For this review, take the finished solid that the model builds, in its own axes (mm). Give positions to 0.01 mm unless a question says otherwise; leave off trailing zeros. Loops run counter-clockwise (first coordinate to the right, second up) from the corner with the lowest first, then second, coordinate; pieces in that order, holes last. Notation, with made-up numbers: (-26.75, 42.25) - (28.25, 42.25) arc R16 cw to (28.25, 49.25) - close; hole circle Ø7 at (87, 82.25). An arc over 180 degrees is marked (long way). Put each result on its own line as item: value. Start each with the question number.
from build123d import *

# Parameters (mm, degrees)
SKETCH1_R            = 15
BOSS_EXTRUDE1_DEPTH  = 1.5875
M5_CLEARANCE_HOLE1_D = 5.8
FILLET1_R            = 10


with BuildPart() as part:
    # Sketch1 → Boss-Extrude1 (new body)
    with BuildSketch(Plane.XY):
        with BuildLine():
            Line((-31.721304871, -10.769995549), (-31.721304871, -61.809795549))
            Line((-31.721304871, -61.809795549), (-244.957511762, -61.809795549))
            Line((-244.957511762, -61.809795549), (-244.957511762, 103.169804451))
            Line((-244.957511762, 103.169804451), (335.042488238, 103.169804451))
            Line((335.042488238, 103.169804451), (335.042488238, -61.809795549))
            Line((335.042488238, -61.809795549), (23.278695129, -61.809795549))
            Line((23.278695129, -61.809795549), (23.278695129, -10.769995549))
            ThreePointArc((23.278695129, -10.769995549), (-4.221304871, 16.730004451), (-31.721304871, -10.769995549))
        make_face()
        with Locations((41.778695129, 44.230004451)):
            Circle(SKETCH1_R, mode=Mode.SUBTRACT)
    extrude(amount=BOSS_EXTRUDE1_DEPTH)

    # M5 Clearance Hole1 (through all)
    with Locations(Plane.XY.offset(1.5875)):
        with Locations((-204.957511762, 93.169804451), (-204.957511762, -51.809795549), (88.121775735, -51.809795549), (295.042488238, -51.809795549), (-84.957511762, 93.169804451), (175.042488238, 93.169804451), (295.042488238, 93.169804451)):
            Hole(M5_CLEARANCE_HOLE1_D / 2)

    # Fillet1
    fillet1_edges = [part.edges().sort_by_distance(p)[0] for p in [
        (-244.957511762, 103.169804451, 0.79375),
        (335.042488238, 103.169804451, 0.79375),
        (335.042488238, -61.809795549, 0.79375),
        (23.278695129, -61.809795549, 0.79375),
        (-31.721304871, -61.809795549, 0.79375),
        (-244.957511762, -61.809795549, 0.79375),
    ]]
    fillet(fillet1_edges, radius=FILLET1_R)


solid = part.part
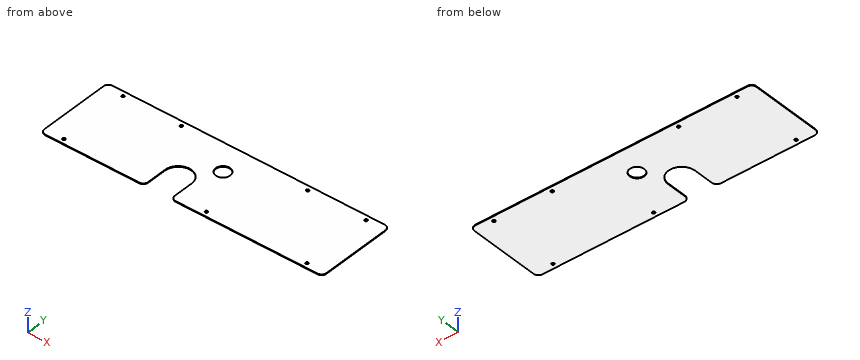
1) Wall thickness on probe 1 along X at (y, z) = (93, 0.9); probe 2 along X at (y, z) = (-18.5, 0.9); probe 3 along Y at (x, z) = (293, 1.2): over which ranges is each line inside the solid? List them lowest first.
2) Take a section at C-C on y = 53. State the section outline as (x, z) points, and give its area (3 significant figures).
3) Take a section at A-A on y = -27. State the section outline as (x, z) points, and give its area (3 significant figures).
4) Take a section at B-B on z = 0.3. State how many separate pieces and enclosed holes the cut face has, and give its area (3 significant figures).
Answers follow:
1. probe 1: -244.96 to -207.85, -202.06 to -87.85, -82.06 to 172.15, 177.94 to 292.15, 297.94 to 335.04
1. probe 2: -244.96 to -31.72, 23.28 to 335.04
1. probe 3: -61.81 to -53.87, -49.75 to 91.11, 95.23 to 103.17
2. outline: (-244.96, 0) - (29.61, 0) - (29.61, 1.59) - (-244.96, 1.59) - close; (53.95, 0) - (335.04, 0) - (335.04, 1.59) - (53.95, 1.59) - close
2. area: 882 mm2
3. outline: (-244.96, 0) - (-31.72, 0) - (-31.72, 1.59) - (-244.96, 1.59) - close; (23.28, 0) - (335.04, 0) - (335.04, 1.59) - (23.28, 1.59) - close
3. area: 833 mm2
4. separate pieces: 1
4. enclosed holes: 8
4. area: 90,700 mm2
